```python
from build123d import *
from OCP.BRepFilletAPI import BRepFilletAPI_MakeChamfer

# Parameters (mm, degrees)
SKETCH_1_W          = 85
SKETCH_1_H          = 90
EXTRUDE_1_DEPTH     = 2.5
CHAMFER_1_SIZE      = 20
CHAMFER_1_SIZE2     = 34.641016151
SKETCH_2_R          = 2.1
CUT_EXTRUDE_1_DEPTH = 172.263685585
FILLET_1_R          = 3
CHAMFER_2_SIZE      = 4
CHAMFER_2_SIZE2     = 4.564598072
CHAMFER_3_SIZE      = 2
CUT_EXTRUDE_3_DEPTH = 172.263685585
CHAMFER_4_SIZE      = 4
FILLET_3_R          = 1


with BuildPart() as part:
    # 草图1 → 凸台-拉伸1 (new, symmetric)
    with BuildSketch(Plane.XY):
        Polygon((-82.5, -150), (82.5, -150), (82.5, -130), (62.5, 40), (-62.5, 40), (-82.5, -130), align=None)
        with Locations((0, -85)):
            Rectangle(SKETCH_1_W, SKETCH_1_H, mode=Mode.SUBTRACT)
    extrude(amount=EXTRUDE_1_DEPTH, both=True)

    # 倒角1
    chamfer_1_edges = [part.edges().sort_by_distance(p)[0] for p in [
        (-42.5, -130, 0),
        (42.5, -130, 0),
    ]]
    chamfer_1_side = [part.faces().sort_by_distance(p)[0] for p in [
        (0, -130, 0),
    ]]
    chamfer(chamfer_1_edges, length=CHAMFER_1_SIZE, length2=CHAMFER_1_SIZE2, reference=chamfer_1_side[0])

    # 草图2 → 切除-拉伸1 (cut, through all)
    with BuildSketch(Plane.XY.offset(2.5)):
        with Locations((-72.5, -140)):
            Circle(SKETCH_2_R)
        with Locations((-32.5, -140)):
            Circle(SKETCH_2_R)
        with Locations((-52.5, 30)):
            Circle(SKETCH_2_R)
        with Locations((-52.5, 10)):
            Circle(SKETCH_2_R)
        with Locations((-52.5, -100)):
            Circle(SKETCH_2_R)
        with Locations((-52.5, -120)):
            Circle(SKETCH_2_R)
        with Locations(Location((52.5, 30, 0), (0, 0, 180))):
            Circle(SKETCH_2_R)
        with Locations(Location((52.5, 10, 0), (0, 0, 180))):
            Circle(SKETCH_2_R)
        with Locations(Location((52.5, -100, 0), (0, 0, 180))):
            Circle(SKETCH_2_R)
        with Locations(Location((52.5, -120, 0), (0, 0, 180))):
            Circle(SKETCH_2_R)
        with Locations(Location((32.5, -140, 0), (0, 0, 180))):
            Circle(SKETCH_2_R)
        with Locations(Location((72.5, -140, 0), (0, 0, 180))):
            Circle(SKETCH_2_R)
    extrude(amount=-CUT_EXTRUDE_1_DEPTH, mode=Mode.SUBTRACT)

    # 圆角1
    fillet_1_edges = [part.edges().sort_by_distance(p)[0] for p in [
        (-42.5, -40, 0),
        (42.5, -40, 0),
        (-22.5, -130, 0),
        (22.5, -130, 0),
        (42.5, -95.358983849, 0),
        (-42.5, -95.358983849, 0),
    ]]
    fillet(fillet_1_edges, radius=FILLET_1_R)

    # 倒角2: one chamfer whose edges measure the first distance from different faces: ONE call of the kernel's chamfer builder (chamfer() names one face for all edges)
    chamfer_2_edges_1 = [part.edges().sort_by_distance(p)[0] for p in [
        (-62.5, 40, 0),
        (62.5, 40, 0),
    ]]
    chamfer_2_side_1 = [part.faces().sort_by_distance(p)[0] for p in [
        (0, 40, 0),
    ]]
    chamfer_2_edges_2 = [part.edges().sort_by_distance(p)[0] for p in [
        (82.5, -150, 0),
        (-82.5, -150, 0),
    ]]
    chamfer_2 = BRepFilletAPI_MakeChamfer(part.part.solid().wrapped)
    for e in chamfer_2_edges_1:
        chamfer_2.Add(CHAMFER_2_SIZE, CHAMFER_2_SIZE2, e.wrapped, chamfer_2_side_1[0].wrapped)  # the first distance lies on this face
    for e in chamfer_2_edges_2:
        chamfer_2.Add(CHAMFER_2_SIZE, e.wrapped)
    add(Compound.cast(chamfer_2.Shape()), mode=Mode.REPLACE)

    # 倒角3
    chamfer_3_edges = [part.edges().sort_by_distance(p)[0] for p in [
        (-74.6, -140, 2.5),
        (74.6, -140, 2.5),
        (34.6, -140, 2.5),
        (54.6, -120, 2.5),
        (-54.6, -100, 2.5),
        (-54.6, 10, 2.5),
        (-54.6, 30, 2.5),
        (-34.6, -140, 2.5),
        (54.6, -100, 2.5),
        (54.6, 10, 2.5),
        (54.6, 30, 2.5),
        (-54.6, -120, 2.5),
    ]]
    chamfer(chamfer_3_edges, length=CHAMFER_3_SIZE)

    # 草图4 → 切除-拉伸3 (cut, through all)
    with BuildSketch(Plane(origin=(0, 0, -2.5), x_dir=(-1, 0, 0), z_dir=(0, 0, -1))):
        Polygon((0, -17.5), (-32.5, -17.5), (-32.5, 17.5), (0, 17.5), (32.5, 17.5), (32.5, -17.5), align=None)
    extrude(amount=-CUT_EXTRUDE_3_DEPTH, mode=Mode.SUBTRACT)

    # 倒角4
    chamfer_4_edges = [part.edges().sort_by_distance(p)[0] for p in [
        (32.5, -17.5, 0),
        (32.5, 17.5, 0),
        (-32.5, 17.5, 0),
        (-32.5, -17.5, 0),
    ]]
    chamfer(chamfer_4_edges, length=CHAMFER_4_SIZE)

    # 圆角3
    fillet_3_edges = [part.edges().sort_by_distance(p)[0] for p in [
        (-32.5, 13.5, 0),
        (-32.5, -13.5, 0),
        (28.5, -17.5, 0),
        (-28.5, -17.5, 0),
        (28.5, 17.5, 0),
        (-28.5, 17.5, 0),
        (32.5, 13.5, 0),
        (32.5, -13.5, 0),
    ]]
    fillet(fillet_3_edges, radius=FILLET_3_R)


solid = part.part
```
Source: CAD feature listing. Evaluate the final solid. Frame: model axes, mm. A direction names the side the tool comes from. Round coordinates to 2 decimals unless told otherwise and drop trailing zeros. Loops run counter-clockwise (first coordinate to the right, second up) from the corner with the lowest first, then second, coordinate; pieces in that order, holes last. Notation, with made-up numbers: (-29, 77) - (29, 77) arc R28 cw to (29, 115) - close; hole circle Ø10 at (-4.5, 52). An arc over 180 degrees is marked (long way). Use CSV: the item, a comma, the result in double quotes.
Q1. Pin query (flat end, axial travel): pin 1 Ø1.5 at (y, z) = (-1, -0.5) entering from -X; pin 2 Ø4 at (x, y) = (32.5, -140) entering from -Z; pin 3 Ø2.5 at (y, z) = (-57.5, -0.5) entering from +X; pin 4 Ø1 at (y, z) = (-7.5, 1.5) entering from +X. Return the tip coordinate at first contact, or that it passes through.
Reported:
pin 1,"x = -67.41"
pin 2,"through"
pin 3,"x = 74.12"
pin 4,"x = 68.15"
Q2. Section query D-D, the plane y = -69. Output: boundary loops of the cut face in (x, z), then the cut area to 3 significant figures.
Reported:
outline,"(-75.32, -2.5) - (-42.5, -2.5) - (-42.5, 2.5) - (-75.32, 2.5) - close; (42.5, -2.5) - (75.32, -2.5) - (75.32, 2.5) - (42.5, 2.5) - close"
area,"328 mm^2"
Q3. Section query A-A, the plane x = 52.5. Output: boundary loops of the cut face in (y, z).
Reported:
outline,"(-150, -2.5) - (-122.1, -2.5) - (-122.1, 0.5) - (-124.1, 2.5) - (-150, 2.5) - close; (-117.9, -2.5) - (-102.1, -2.5) - (-102.1, 0.5) - (-104.1, 2.5) - (-115.9, 2.5) - (-117.9, 0.5) - close; (-97.9, -2.5) - (7.9, -2.5) - (7.9, 0.5) - (5.9, 2.5) - (-95.9, 2.5) - (-97.9, 0.5) - close; (12.1, -2.5) - (27.9, -2.5) - (27.9, 0.5) - (25.9, 2.5) - (14.1, 2.5) - (12.1, 0.5) - close; (32.1, -2.5) - (40, -2.5) - (40, 2.5) - (34.1, 2.5) - (32.1, 0.5) - close"
Q4. Reachability of faces 1 (the flat face through (-1, -40, 0)), 2 (the flat face through (1, 40, 0)) from +Z, -Z, +X, -X, +Y, -Y: full face, straight path, thin tool, end or side. Return the list, or none.
Reported:
face 1,"+Z, -Z"
face 2,"+Z, -Z, +X, -X, +Y"
Q5. Ray query, line 1 along Y through (x, z) = (-52.5, -0.4); line 2 along Y through (x, z) = (0, -1.45); line 3 along Y through (x, z) = (51.5, -1.4). Return the intervals inside material, ascending.
Reported:
line 1,"-150 to -122.1, -117.9 to -102.1, -97.9 to 7.9, 12.1 to 27.9, 32.1 to 40"
line 2,"-150 to -130, -40 to -17.5, 17.5 to 40"
line 3,"-150 to -121.85, -118.15 to -101.85, -98.15 to 8.15, 11.85 to 28.15, 31.85 to 40"
Q6. Section query B-B, the plane y = -140. Output: boundary loops of the cut face in (x, z).
Reported:
outline,"(-82.5, -2.5) - (-74.6, -2.5) - (-74.6, 0.5) - (-76.6, 2.5) - (-82.5, 2.5) - close; (-70.4, -2.5) - (-34.6, -2.5) - (-34.6, 0.5) - (-36.6, 2.5) - (-68.4, 2.5) - (-70.4, 0.5) - close; (-30.4, -2.5) - (30.4, -2.5) - (30.4, 0.5) - (28.4, 2.5) - (-28.4, 2.5) - (-30.4, 0.5) - close; (34.6, -2.5) - (70.4, -2.5) - (70.4, 0.5) - (68.4, 2.5) - (36.6, 2.5) - (34.6, 0.5) - close; (74.6, -2.5) - (82.5, -2.5) - (82.5, 2.5) - (76.6, 2.5) - (74.6, 0.5) - close"
Q7. Section query C-C, the plane x = 72.5. Output: boundary loops of the cut face in (y, z), then the cut area to 3 significant figures.
Reported:
outline,"(-150, -2.5) - (-142.1, -2.5) - (-142.1, 0.5) - (-144.1, 2.5) - (-150, 2.5) - close; (-137.9, -2.5) - (-45, -2.5) - (-45, 2.5) - (-135.9, 2.5) - (-137.9, 0.5) - close"
area,"500 mm^2"
Q8. Mould query, pull axis X, two halves, no side actions, for faces 3 (the cylindrical face through (34.6, -140.09, -0.98)), 4 (the flat face through (82.5, -138, 0)), 5 (the flat face through (-80.5, -148, 0)). Classes: pulls with the +X half, pulls with the -X half, needs draft (parallel to the pull), parting line crosses it, or undercut.
Reported:
face 3,"undercut"
face 4,"pulls with the +X half"
face 5,"pulls with the -X half"
